Study the drawing (mm; zero at the part's minimum x, y, z) and answer. Coordinates: 2 decimals unless noted, no trailing zeros. Order: outer loops, then holes, each group sorted by start corner. A loop starts at its lowest first (then second) coordinate and runs counter-clockwise, first axis right, second up. Notation, with made-up numbers: M -12,80.5 L 7,80.5 A26 cw 7,106.5 Z; hole C -36,-29.75 d11. An arc over 180 degrees is marked long. Put each result on its own line as item: value.
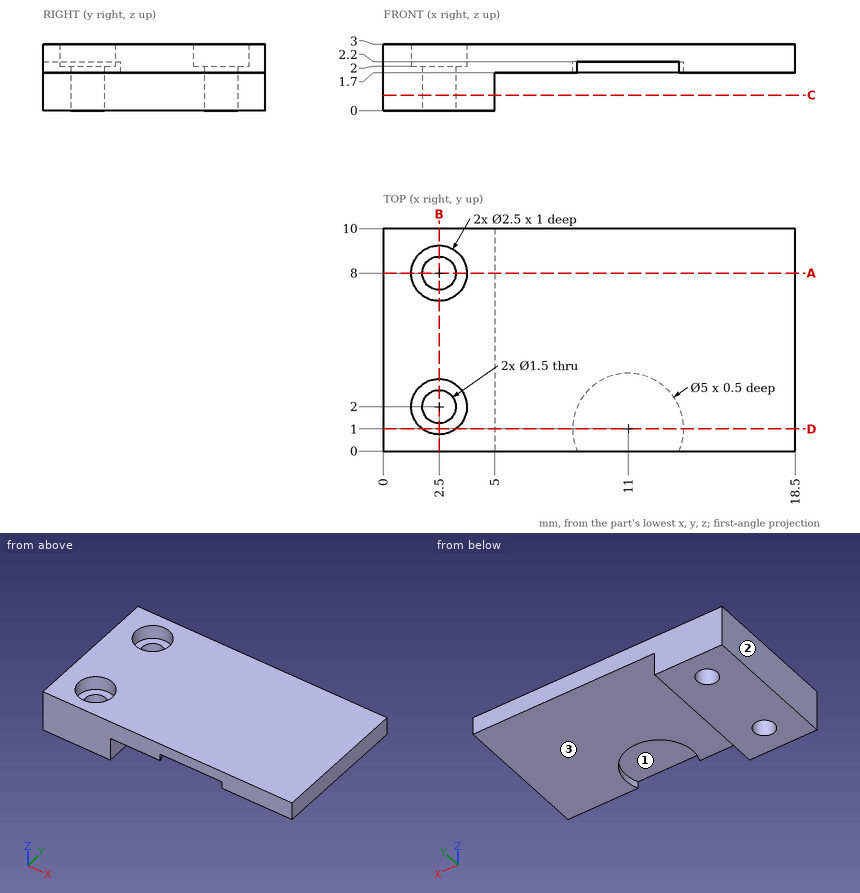
Q1. Find section A-A on y = 8. Write down the section's boundary in (x, z), plus the area to 4 significant figures.
Answers below:
outline: M 0,0 L 1.75,0 L 1.75,2 L 1.25,2 L 1.25,3 L 0,3 Z; M 3.25,0 L 5,0 L 5,1.7 L 18.5,1.7 L 18.5,3 L 3.75,3 L 3.75,2 L 3.25,2 Z
area: 27.05 mm^2
Q2. For a pull along X with two mould halves and no side action, classify the marked faces 1, 2 and 3 as +X half, -X half, draft (parallel to the pull), parting line (faces both ways), or undercut.
Answers below:
face 1: undercut
face 2: -X half
face 3: draft
Q3. Find section C-C on z = 0.7. Write down the section's boundary in (x, y), plus the area to 3 significant figures.
Answers below:
outline: M 0,0 L 5,0 L 5,10 L 0,10 Z; hole C 2.5,2 d1.5; hole C 2.5,8 d1.5
area: 46.5 mm^2
Q4. Find section D-D on y = 1. Write down the section's boundary in (x, z).
Answers below:
outline: M 0,0 L 5,0 L 5,1.7 L 8.5,1.7 L 8.5,2.2 L 13.5,2.2 L 13.5,1.7 L 18.5,1.7 L 18.5,3 L 3.25,3 L 3.25,2 L 1.75,2 L 1.75,3 L 0,3 Z
Q5. Given pin 1 (0.5 mm diameter, centred on y = 4, z = 1, fed in from +X); pin 2 (1.5 mm diameter, centred on x = 14.5, y = 5, fed in from -Z); pin 3 (0.8 mm diameter, centred on x = 3, y = 1.5, fed in from +Z), each flat-ended and moving along its own axis, determine where each tip first touches the part or whether it passes through.
Answers below:
pin 1: stops at x = 5
pin 2: stops at z = 1.7
pin 3: stops at z = 2
Q6. Find section B-B on x = 2.5. Write down the section's boundary in (y, z).
Answers below:
outline: M 0,0 L 1.25,0 L 1.25,2 L 0.75,2 L 0.75,3 L 0,3 Z; M 2.75,0 L 7.25,0 L 7.25,2 L 6.75,2 L 6.75,3 L 3.25,3 L 3.25,2 L 2.75,2 Z; M 8.75,0 L 10,0 L 10,3 L 9.25,3 L 9.25,2 L 8.75,2 Z
Q7. Consider line 1 along Y through (x, z) = (2.5, 0.75); line 2 along Y through (x, z) = (2.5, 2.75); line 3 along X through (y, z) = (1.5, 1.8). Determine where each line is inside the solid, lowest interval first.
Answers below:
line 1: y = 0 to 1.25, 2.75 to 7.25, 8.75 to 10
line 2: y = 0 to 0.75, 3.25 to 6.75, 9.25 to 10
line 3: x = 0 to 1.94, 3.06 to 8.55, 13.45 to 18.5
